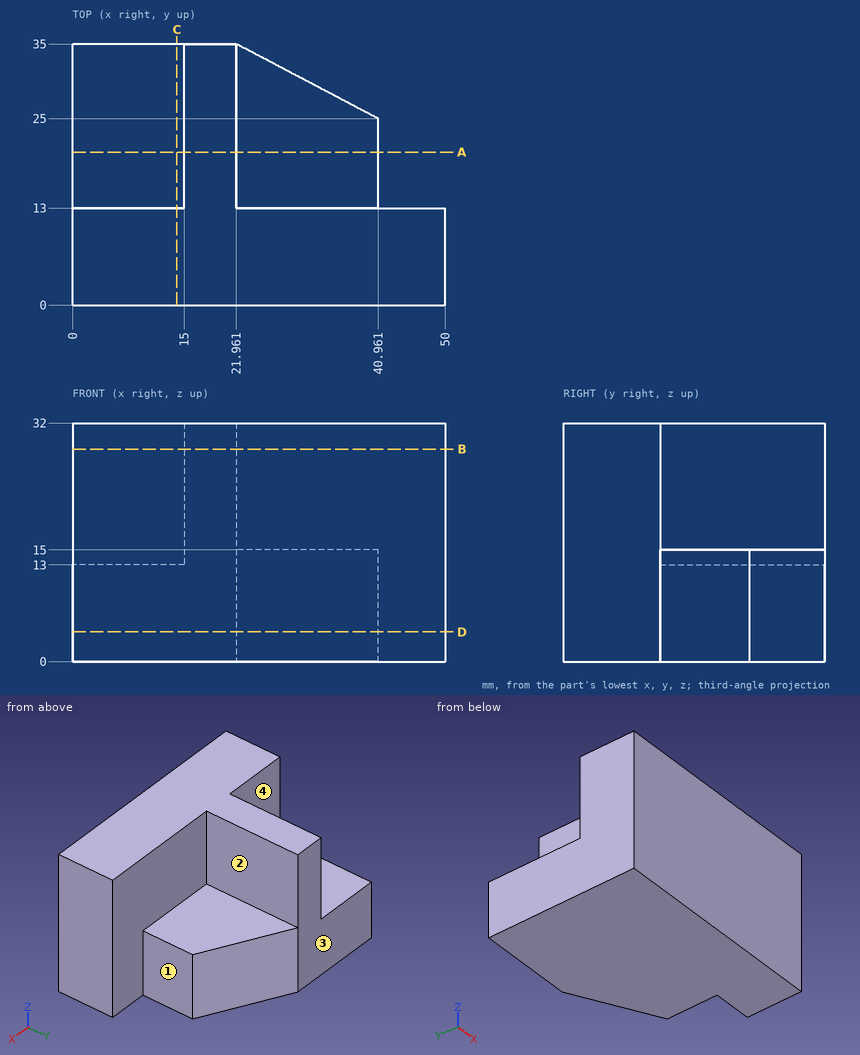
Print and shaded views of the part. All mm, measured from the part's lowest x, y and z. A direction names the side the tool comes from. Round coordinates to 2 decimals unless told otherwise and drop trailing zeros. Loops run counter-clockwise (first coordinate to the right, second up) from the corner with the lowest first, then second, coordinate; pieces in that order, holes last. Notation, with made-up numbers: M -12,11 L 23,11 A23 ccw 23,34 Z; hole C 11,74 d10. An arc over 180 degrees is marked long. One line per question, with ' | ' between items.
1) Flat gauge pins, fed straight in: pin 1 (6 mm diameter, centred on y = 20.5, z = 4.5, fed in from +X); pin 2 (7.5 mm diameter, centred on x = 7, z = 19, fed in from +Y); pin 3 (15 mm diameter, centred on x = 34, y = 29, fed in from +Z). Where does each tip first touch, or does it go through?
Solved:
pin 1: stops at x = 40.96 | pin 2: stops at y = 13 | pin 3: stops at z = 15
2) Band-saw the part on D-D (z = 4). Give the cut face in (x, y).
Solved:
outline: M 0,0 L 50,0 L 50,13 L 40.96,13 L 40.96,25 L 21.96,35 L 0,35 Z
3) Drill centre lines: line 1 along Y through (x, z) = (46.5, 25.5); line 2 along X through (y, z) = (31, 29.5); line 3 along X through (y, z) = (15, 3.5). Where is each one in solid material? Low to high.
Solved:
line 1: y = 0 to 13 | line 2: x = 15 to 21.96 | line 3: x = 0 to 40.96
4) Band-saw the part on A-A (y = 20.5). Give the cut face in (x, z).
Solved:
outline: M 0,0 L 40.96,0 L 40.96,15 L 21.96,15 L 21.96,32 L 15,32 L 15,13 L 0,13 Z
5) Band-saw the part on B-B (z = 28.5). Give the cut face in (x, y).
Solved:
outline: M 0,0 L 50,0 L 50,13 L 21.96,13 L 21.96,35 L 15,35 L 15,13 L 0,13 Z
6) Band-saw the part on C-C (x = 14). Give the cut face in (y, z), then the cut area to 3 significant figures.
Solved:
outline: M 0,0 L 35,0 L 35,13 L 13,13 L 13,32 L 0,32 Z | area: 702 mm²
7) 3-axis set-ups, long thin cutter, end or side, ignore diameter. For the marked faces 1, 2, 3 and 4: which of +Z, -Z, +X, -X, +Y, -Y reach the whole face in a straight line?
Solved:
face 1: +Z, -Z, +X, +Y | face 2: +Z, +X, +Y | face 3: +Z, -Z, +X, -X, +Y | face 4: +Z, -X, +Y
